from build123d import *

# Parameters (mm, degrees)
BOSS_EXTRUDE1_DEPTH = 20
SKETCH3_R           = 5
BOSS_EXTRUDE2_DEPTH = 30
FILLET1_R           = 1


with BuildPart() as part:
    # Sketch1 → Boss-Extrude1 (new body, symmetric)
    with BuildSketch(Plane(origin=(0, 0, 0), x_dir=(0, 0, -1), z_dir=(1, 0, 0))):
        with BuildLine():
            Line((5, -8.660254038), (5, -13.660254038))
            Line((5, -13.660254038), (15, -13.660254038))
            Line((15, -13.660254038), (15, 16.339745962))
            Line((15, 16.339745962), (-15, 16.339745962))
            Line((-15, 16.339745962), (-15, -13.660254038))
            Line((-15, -13.660254038), (-5, -13.660254038))
            Line((-5, -13.660254038), (-5, -8.660254038))
            ThreePointArc((-5, -8.660254038), (0, 10), (5, -8.660254038))
        make_face()
    extrude(amount=BOSS_EXTRUDE1_DEPTH, both=True)

    # Sketch3 → Boss-Extrude2 (add)
    with BuildSketch(Plane.XY.offset(15)):
        with BuildLine():
            Line((-20, 16.339745962), (20, 16.339745962))
            Line((20, 16.339745962), (4.931506849, 29.490430894))
            ThreePointArc((4.931506849, 29.490430894), (0, 31.339745962), (-4.931506849, 29.490430894))
            Line((-4.931506849, 29.490430894), (-20, 16.339745962))
        make_face()
        with Locations((0, 23.839745962)):
            Circle(SKETCH3_R, mode=Mode.SUBTRACT)
    extrude(amount=-BOSS_EXTRUDE2_DEPTH)

    # Fillet1
    fillet1_edges = [part.edges().sort_by_distance(p)[0] for p in [
        (20, -13.660254038, -10),
        (-20, -11.160254038, -5),
        (-20, 10, 0),
        (20, 1.339745962, -15),
        (0, -13.660254038, 5),
        (0, -13.660254038, 15),
        (0, -13.660254038, -15),
        (0, -13.660254038, -5),
        (20, 16.339745962, 0),
        (20, 1.339745962, 15),
        (20, -13.660254038, 10),
        (-12.465753425, 22.915088428, 15),
        (12.465753425, 22.915088428, 15),
        (0, 31.339745962, 15),
        (20, -11.160254038, 5),
        (-12.465753425, 22.915088428, -15),
        (0, 31.339745962, -15),
        (12.465753425, 22.915088428, -15),
        (20, 10, 0),
        (20, -11.160254038, -5),
        (-20, -11.160254038, 5),
        (-20, -13.660254038, 10),
        (-20, 1.339745962, 15),
        (-20, 16.339745962, 0),
        (-20, 1.339745962, -15),
        (-20, -13.660254038, -10),
    ]]
    fillet(fillet1_edges, radius=FILLET1_R)


solid = part.part
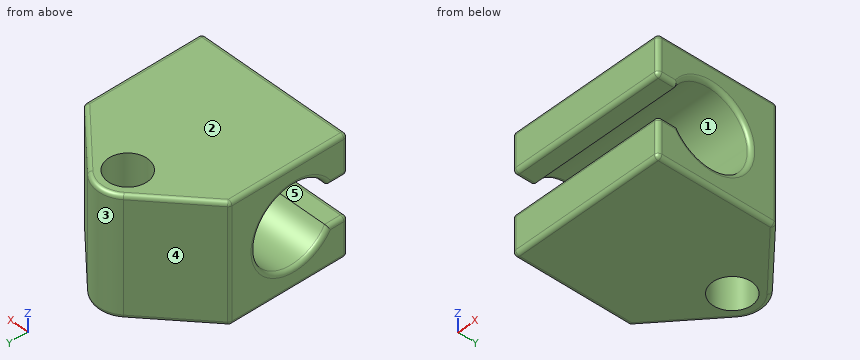
Input: part model. Units: mm. Frame: model coordinates. Face numbers are marked on the shaded views. A direction names the side the tool comes from. Round coordinates to 2 decimals unless told otherwise and drop trailing zeros. Order: outer loops, then holes, each group sorted by start corner. A loop starts at its lowest first (then second) coordinate and runs counter-clockwise, first axis right, second up.
1. Material intervals for line 1 (Y direction, x = 4, z = 6); line 2 (Y direction, x = 0, z = -8.25); line 3 (Z direction, x = -7, y = 0), sorted ascending.
The answers:
line 1: y = -13.66 to -8, 8 to 20.84, 26.84 to 30.18
line 2: y = -13.66 to -5.65, 5.65 to 18.84, 28.84 to 31.34
line 3: z = -15 to -10, 10 to 15
2. Mould query, pull axis Z, two halves, no side actions, for the marked faces 1, 2 and 3. Classes: released by +Z, released by -Z, zero draft, split by the parting line, or undercut.
The answers:
face 1: undercut
face 2: released by +Z
face 3: zero draft
3. Cut plane D-D, the plane z = 13. Output: boundary loops of the cut face in (x, y), then the cut area to 3 significant figures.
The answers:
outline: (-20, -12.66) arc R1 ccw to (-19, -13.66) - (19, -13.66) arc R1 ccw to (20, -12.66) - (20, 15.89) arc R1 ccw to (19.66, 16.64) - (4.93, 29.49) arc R7.5 ccw to (-4.93, 29.49) - (-19.66, 16.64) arc R1 ccw to (-20, 15.89) - close; hole circle Ø10 at (0, 23.84)
area: 1,460 mm2
4. Cut plane C-C, the plane z = 0. Output: boundary loops of the cut face in (x, y).
The answers:
outline: (-20, 11) arc R1 ccw to (-19, 10) - (19, 10) arc R1 ccw to (20, 11) - (20, 15.89) arc R1 ccw to (19.66, 16.64) - (4.93, 29.49) arc R7.5 ccw to (-4.93, 29.49) - (-19.66, 16.64) arc R1 ccw to (-20, 15.89) - close; hole circle Ø10 at (0, 23.84)
5. Set-up query: the marked faces 4 and 5. Return all of +Z, -Z, +X, -X, +Y, -Y with unobstructed straight access to the full face (end or side cutting, diameter ignored); none if empty.
The answers:
face 4: +Z, -Z, -X, +Y
face 5: +X, -X, -Y
6. Cut plane B-B, the plane z = 7.5. State how many separate pieces and enclosed holes the cut face has, then the cut area to 3 significant figures.
The answers:
separate pieces: 2
enclosed holes: 1
area: 931 mm2
7. Cut plane A-A, the plane x = 0. Output: boundary loops of the cut face in (y, z), then the cut area to 3 significant figures.
The answers:
outline: (-13.66, -14) arc R1 ccw to (-12.66, -15) - (18.84, -15) - (18.84, 15) - (-12.66, 15) arc R1 ccw to (-13.66, 14) - (-13.66, 6) arc R1 ccw to (-12.66, 5) - (-8.66, 5) arc R10 cw (long way) to (-8.66, -5) - (-12.66, -5) arc R1 ccw to (-13.66, -6) - close; (28.84, -15) - (30.34, -15) arc R1 ccw to (31.34, -14) - (31.34, 14) arc R1 ccw to (30.34, 15) - (28.84, 15) - close
area: 694 mm2
